Autodesk Fusion 360 part; units mm, degrees
sketch "Sketch1" plane through (0, 0, 0) normal (0, 1, 0) x (1, 0, 0)
  line L0 (0, 0) -> (33.5, 0)
  circle A0 centre (0, 0) radius 1.75
  circle A1 centre (33.5, 0) radius 1.75
  circle A2 centre (33.5, 0) radius 4
  circle A3 centre (0, 0) radius 4
  line L1 (0, 4) -> (33.5, 4)
  line L2 (33.5, -4) -> (0, -4)
  dimension "d1" = 33.5
  dimension "d2" = 3.5
  dimension "d3" = 3.5
  dimension "d4" = 8
  dimension "d5" = 8
extrude "Extrude1" add sketch "Sketch1" along normal blind 3 makes body 1
hole "Hole1" at (0, 3, 0) direction (0, -1, 0) diameter 5 depth 1.5 tip angle 118 bodies 1
hole "Hole2" at (33.5, 3, 0) direction (0, -1, 0) diameter 5 depth 1.5 tip angle 118 bodies 1
sketch "Sketch9" plane through (0, 3, 0) normal (0, 1, 0) x (-1, 0, 0)
  circle A0 centre (-33.5, 0) radius 2.5
  circle A1 centre (0, 0) radius 2.5
  arc A2 (0, -4) -> (0, 4) centre (0, 0) ccw
  line L0 (0, 4) -> (-33.5, 4)
  arc A3 (-33.5, 4) -> (-33.5, -4) centre (-33.5, 0) ccw
  line L1 (-33.5, -4) -> (0, -4)
  line L2 (-16.75, 4) -> (-5.75, 4)
  line L3 (-16.75, 4) -> (-27.75, 4)
  line L4 (-27.75, 4) -> (-27.75, -4)
  line L5 (-5.75, 4) -> (-5.75, -4)
  circle A4 centre (0, 0) radius 5
  circle A5 centre (-33.5, 0) radius 5
  dimension "d79" = 11
  dimension "d80" = 11
  dimension "d81" = 10
  dimension "d82" = 10
extrude "Extrude13" add sketch "Sketch9" along normal blind 4 contours L0 L1 L5 A4 | L0 L1 L4 A5 bodies 1
extrude "Extrude14" cut sketch "Sketch9" against normal blind 3 contours L0 L1 L2 L3 L4 L5 bodies 1 makes body 2 at (2.2804, 0, -3.1227)
sketch "Sketch10" plane through (5.75, 0, 0) normal (1, 0, 0) x (0, 0, -1)
  line L0 (4, 0) -> (4, 7)
  line L1 (4, 7) -> (-4, 7)
  line L2 (-4, 7) -> (-4, 0)
  line L3 (-4, 0) -> (4, 0)
  line L4 (-4, 7) -> (4, 7)
  line L5 (4, 7) -> (4, 4)
  line L6 (4, 4) -> (-4, 4)
  line L7 (-4, 4) -> (-4, 7)
  dimension "d87" = 3
extrude "Extrude15" add sketch "Sketch10" along normal blind 22 contours L0 L1 L2 L4 L5 L6 L7 bodies 1 2
sketch "Sketch11" plane through (0, 0, 4) normal (0, 0, 1) x (1, 0, 0)
  line L0 (30.5, 7) -> (3, 7)
  line L1 (3, 7) -> (3, 3)
  line L2 (33.5, 3) -> (30.5, 3)
  line L3 (0, 3) -> (0, 0)
  line L4 (27.75, 0) -> (33.5, 0)
  line L5 (5.75, 0) -> (5.75, 4)
  line L6 (5.75, 4) -> (27.75, 4)
  line L7 (5.75, 4) -> (3, 4)
  line L8 (3, 4) -> (6, 4)
  arc A0 (6, 7) -> (3, 4) centre (6, 4) ccw
  line L9 (27.75, 4) -> (27.75, 0)
  line L10 (33.5, 0) -> (33.5, 3)
  line L11 (30.5, 3) -> (30.5, 7)
  line L12 (3, 3) -> (0, 3)
  line L13 (0, 0) -> (5.75, 0)
  line L14 (30.5, 4) -> (27.5, 4)
  arc A1 (30.5, 4) -> (27.5, 7) centre (27.5, 4) ccw
  dimension "d90" = 3
  dimension "d101" = 3
extrude "Extrude16" cut sketch "Sketch11" against normal blind 10 contours L0 L11 A1 | L0 L1 A0 bodies 1
sketch "Sketch12" plane through (0, 0, 4) normal (0, 0, 1) x (1, 0, 0)
  line L0 (27.75, 4) -> (27.75, 0)
  line L1 (0, 0) -> (5.75, 0)
  line L2 (33.5, 0) -> (33.5, 3)
  line L3 (3, 3) -> (0, 3)
  line L4 (30.5, 3) -> (30.5, 4)
  line L5 (27.5, 7) -> (6, 7)
  line L6 (27.75, 4) -> (24.75, 4)
  line L7 (24.75, 4) -> (24.75, 1)
  arc A0 (27.75, 1) -> (24.75, 4) centre (24.75, 1) ccw
  arc A1 (6, 7) -> (3, 4) centre (6, 4) ccw
  line L8 (3, 4) -> (3, 3)
  line L9 (0, 3) -> (0, 0)
  line L10 (5.75, 0) -> (5.75, 4)
  line L11 (5.75, 4) -> (27.75, 4)
  arc A2 (30.5, 4) -> (27.5, 7) centre (27.5, 4) ccw
  line L12 (27.75, 0) -> (33.5, 0)
  line L13 (33.5, 3) -> (30.5, 3)
  line L14 (5.75, 4) -> (8.75, 4)
  line L15 (8.75, 4) -> (8.75, 1)
  arc A3 (8.75, 4) -> (5.75, 1) centre (8.75, 1) ccw
  dimension "d94" = 3
  dimension "d95" = 3
  dimension "d102" = 3
  dimension "d103" = 3
extrude "Extrude17" add sketch "Sketch12" against normal blind 8 contours L0 L6 A0 L11 | L10 L11 L14 A3 bodies 1
Geometry: final body of the model. Coordinates: model frame, mm. A direction names the side the tool comes from. Coordinates: 2 decimals unless noted, no trailing zeros. Write each loop counter-clockwise with the first axis right and the second up, starting at its lowest first coordinate (ties: lowest second). Pieces come first, ordered by that corner, then holes. Notation, with made-up numbers: M -5.75,-25 L 51.25,-25 A22 cw 51.25,2 Z; hole C 79.25,13 d10. An arc over 180 degrees is marked long. Answer as CSV lines item,"result". Start each with the question number.
Q1. Reachability of faces 4 (the cylindrical face through (28.5, 4.9, 0.1)), 5 (the cylindrical face through (6.65, 3.14, 0.06)), 6 (the flat face through (2, 3, 2)), 7 (the cylindrical face through (2.44, 2.24, -0.54)) from +Z, -Z, +X, -X, +Y, -Y: full face, straight path, thin tool, end or side. Return the list, or none.
Q2. Cut plane D-D on y = 5.25. Return the cut outline in (x, z).
Q3. Mould query, pull axis Z, two halves, no side actions, for faces 1 (the flat face through (16.5, 4.2, -4)), 2 (the flat face through (5.75, 0.5, 0.1)), 3 (the cylindrical face through (5, 5, 0)). Classes: released by +Z, released by -Z, zero draft, split by the parting line, or undercut.
Q4. Line query: line 1 (X direction, y = 2.2, z = 0); line 2 (X direction, y = 0.5, z = 0); line 3 (Y direction, x = 13.5, z = 1.5). Output: solid intervals per line, ascending. Write a range as from..to.
Q5. Pin query (flat end, axial travel): P1, Ø2.5, axis at x = 18, z = 0.5, coming from the -Y side; P2, Ø2, axis at y = 1.5, z = -2.5, coming from the +X side; P3, Ø3, axis at x = 0, z = 0, coming from the -Y side; P4, Ø4, axis at x = 1, z = 1, coming from the +Y side. Return the tip coordinate at first contact, or that it passes through.
Q6. Cut plane A-A on y = 2. Return the cut outline in (x, z), then the cut area to 3 significant figures.
Q7. Cut plane B-B on z = 0. Count the separate pieces of the cut face and the enclosed holes in it, then the cut area to 3 significant figures.
Q8. Cut plane C-C on x = 29. Return the cut outline in (y, z), then the cut area to 3 significant figures.
Findings below:
1,face 4,"+X, +Y"
1,face 5,"+Z, -Z, -Y"
1,face 6,"-X, +Y"
1,face 7,"+Y"
2,outline,"M 3.27,-4 L 30.23,-4 L 30.23,-3.78 A5 cw 30.23,3.78 L 30.23,4 L 3.27,4 L 3.27,3.78 A5 cw 3.27,-3.78 Z"
3,face 1,"released by -Z"
3,face 2,"zero draft"
3,face 3,"undercut"
4,line 1,"x = -4..-2.5, 2.5..6, 27.5..31, 36..37.5"
4,line 2,"x = -4..-1.75, 1.75..5.75, 27.75..31.75, 35.25..37.5"
4,line 3,"y = 4..7"
5,P1,"stops at y = 4"
5,P2,"stops at x = 37.21"
5,P3,"passes through"
5,P4,"stops at y = 3"
6,outline,"M 0,-4 L 5.92,-4 L 5.92,4 L 0,4 A4 ccw Z; M 27.58,-4 L 33.5,-4 A4 ccw 33.5,4 L 27.58,4 Z; hole C 0,0 d5; hole C 33.5,0 d5"
6,area,"106 mm2"
7,separate pieces,"3"
7,enclosed holes,"0"
7,area,"108 mm2"
8,outline,"M 0,-4 L 6.6,-4 L 6.6,-2.18 L 3,-2.18 L 3,2.18 L 6.6,2.18 L 6.6,4 L 0,4 Z"
8,area,"37.1 mm2"
